```python
from build123d import *

# Parameters (mm, degrees)
PLATE_START        = -27.05
PLATE_B_DEPTH      = 5
PIN_START          = -27.25
SKETCH2_R          = 7.25
PIN_SEATS_DEPTH    = 1.2
BOLT_START         = -27.25
SKETCH3_R          = 1.7
BOLT_HOLES_DEPTH   = 5.4
PIN_START_2        = -24.75
PIN_NUTS_DEPTH     = 2.9
COUNTERBORES_START = -27.25
SKETCH5_R          = 3.2
COUNTERBORES_DEPTH = 3.2


with BuildPart() as part:
    # Sketch1 → Plate B (new body)
    with BuildSketch(Plane(origin=(0, 0, 0), x_dir=(0, 0, -1), z_dir=(1, 0, 0)).offset(PLATE_START)):
        with BuildLine():
            Line((-32, 127.975478406), (-32, 177.024521594))
            ThreePointArc((-32, 177.024521594), (-32.49156491, 179.402996496), (-33.885714286, 181.391746464))
            ThreePointArc((-33.885714286, 181.391746464), (-14, 231.5), (5.885714286, 181.391746464))
            ThreePointArc((5.885714286, 181.391746464), (4.49156491, 179.402996496), (4, 177.024521594))
            Line((4, 177.024521594), (4, 127.975478406))
            ThreePointArc((4, 127.975478406), (4.49156491, 125.597003504), (5.885714286, 123.608253536))
            ThreePointArc((5.885714286, 123.608253536), (-14, 73.5), (-33.885714286, 123.608253536))
            ThreePointArc((-33.885714286, 123.608253536), (-32.49156491, 125.597003504), (-32, 127.975478406))
        make_face()
    extrude(amount=PLATE_B_DEPTH)

    # Sketch2 → Pin seats (cut)
    with BuildSketch(Plane(origin=(0, 0, 0), x_dir=(0, 0, -1), z_dir=(1, 0, 0)).offset(PIN_START)):
        with Locations((-14, 102.5)):
            Circle(SKETCH2_R)
        with Locations((-14, 202.5)):
            Circle(SKETCH2_R)
    extrude(amount=PIN_SEATS_DEPTH, mode=Mode.SUBTRACT)

    # Sketch3 → Bolt holes (cut)
    with BuildSketch(Plane(origin=(0, 0, 0), x_dir=(0, 0, -1), z_dir=(1, 0, 0)).offset(BOLT_START)):
        with Locations((-14, 102.5)):
            Circle(SKETCH3_R)
        with Locations((-14, 202.5)):
            Circle(SKETCH3_R)
        with Locations((0, 122.5)):
            Circle(SKETCH3_R)
        with Locations((-28, 122.5)):
            Circle(SKETCH3_R)
        with Locations((0, 157.5)):
            Circle(SKETCH3_R)
        with Locations((-28, 157.5)):
            Circle(SKETCH3_R)
        with Locations((0, 202.5)):
            Circle(SKETCH3_R)
        with Locations((-28, 202.5)):
            Circle(SKETCH3_R)
    extrude(amount=BOLT_HOLES_DEPTH, mode=Mode.SUBTRACT)

    # Sketch4 → Pin nuts (cut)
    with BuildSketch(Plane(origin=(0, 0, 0), x_dir=(0, 0, -1), z_dir=(1, 0, 0)).offset(PIN_START_2)):
        Polygon((-15.703183294, 105.45), (-17.406366588, 102.5), (-15.703183294, 99.55), (-12.296816706, 99.55), (-10.593633412, 102.5), (-12.296816706, 105.45), align=None)
        Polygon((-15.703183294, 205.45), (-17.406366588, 202.5), (-15.703183294, 199.55), (-12.296816706, 199.55), (-10.593633412, 202.5), (-12.296816706, 205.45), align=None)
    extrude(amount=PIN_NUTS_DEPTH, mode=Mode.SUBTRACT)

    # Sketch5 → Counterbores (cut)
    with BuildSketch(Plane(origin=(0, 0, 0), x_dir=(0, 0, -1), z_dir=(1, 0, 0)).offset(COUNTERBORES_START)):
        with Locations((0, 122.5)):
            Circle(SKETCH5_R)
        with Locations((-28, 122.5)):
            Circle(SKETCH5_R)
        with Locations((0, 157.5)):
            Circle(SKETCH5_R)
        with Locations((-28, 157.5)):
            Circle(SKETCH5_R)
        with Locations((0, 202.5)):
            Circle(SKETCH5_R)
        with Locations((-28, 202.5)):
            Circle(SKETCH5_R)
    extrude(amount=COUNTERBORES_DEPTH, mode=Mode.SUBTRACT)


solid = part.part
```
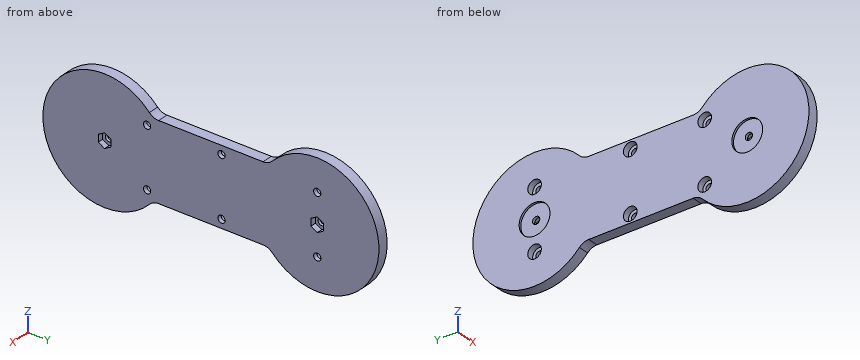
Geometry: final body of the model. Coordinates: model frame, mm. Coordinates: 2 decimals unless noted, no trailing zeros. Order: outer loops, then holes, each group sorted by start corner. A loop starts at its lowest first (then second) coordinate and runs counter-clockwise, first axis right, second up. Notation, with made-up numbers: M 51.5,-8 L 93.5,-8 A21 cw 93.5,30 Z; hole C 21.5,36 d8. An arc over 180 degrees is marked long. Answer as CSV lines item,"result".
Q1. First-contact query: P1, Ø4, axis at y = 202.5, z = 0, coming from the -X side; P2, Ø1, axis at x = -24.5, z = -2.5, coming from the +Y side; P3, Ø1, axis at x = -26, y = 120.5, coming from the -Z side. Flat tips, straight axial feed; report the tip coordinate or a pass-through.
Answers:
P1,"stops at x = -24.05"
P2,"stops at y = 226.69"
P3,"stops at z = -9.12"
Q2. Section B-B on x = -22.9. Count the separate pieces of the cut face and the enclosed holes in it, and give its area (3 significant figures).
Answers:
separate pieces,"1"
enclosed holes,"8"
area,"6,830 mm^2"
Q3. Line query: probe 1 along Y at (x, z) = (-23.65, 15); probe 2 along Z at (x, y) = (-23.05, 202.5); probe 3 along Z at (x, y) = (-23.4, 157.5). Output: solid intervals per line, ascending. Write a range as [from, to].
Answers:
probe 1,"y = [73.52, 99.55], [105.45, 199.55], [205.45, 231.48]"
probe 2,"z = [-15, -1.7], [1.7, 10.59], [17.41, 26.3], [29.7, 43]"
probe 3,"z = [-4, -1.7], [1.7, 26.3], [29.7, 32]"
Q4. Section D-D on z = 38.5. Return the cut outline in (x, y), and give its area (3 significant figures).
Answers:
outline,"M -27.05,86.98 L -22.05,86.98 L -22.05,118.02 L -27.05,118.02 Z; M -27.05,186.98 L -22.05,186.98 L -22.05,218.02 L -27.05,218.02 Z"
area,"310 mm^2"
Q5. Section A-A on z = 14. Return the cut outline in (x, y).
Answers:
outline,"M -27.05,73.5 L -22.05,73.5 L -22.05,99.55 L -24.75,99.55 L -24.75,100.8 L -26.05,100.8 L -26.05,95.25 L -27.05,95.25 Z; M -27.05,109.75 L -26.05,109.75 L -26.05,104.2 L -24.75,104.2 L -24.75,105.45 L -22.05,105.45 L -22.05,199.55 L -24.75,199.55 L -24.75,200.8 L -26.05,200.8 L -26.05,195.25 L -27.05,195.25 Z; M -27.05,209.75 L -26.05,209.75 L -26.05,204.2 L -24.75,204.2 L -24.75,205.45 L -22.05,205.45 L -22.05,231.5 L -27.05,231.5 Z"
Q6. Section C-C on y = 157.5. Return the cut outline in (x, z), and give its area (3 significant figures).
Answers:
outline,"M -27.05,-4 L -22.05,-4 L -22.05,-1.7 L -24.05,-1.7 L -24.05,-3.2 L -27.05,-3.2 Z; M -27.05,3.2 L -24.05,3.2 L -24.05,1.7 L -22.05,1.7 L -22.05,26.3 L -24.05,26.3 L -24.05,24.8 L -27.05,24.8 Z; M -27.05,31.2 L -24.05,31.2 L -24.05,29.7 L -22.05,29.7 L -22.05,32 L -27.05,32 Z"
area,"128 mm^2"
